Part model, mm, in its own coordinate system. A direction names the side the tool comes from. Coordinates: 2 decimals unless noted, no trailing zeros. Loops run counter-clockwise (first coordinate to the right, second up) from the corner with the lowest first, then second, coordinate; pieces in that order, holes last.
Autodesk Inventor part; units mm, degrees
ref_plane "YZ Plane" through (0, 0, 0) normal (1, 0, 0) x (0, 1, 0)
ref_plane "XZ Plane" through (0, 0, 0) normal (0, 1, 0) x (-1, 0, 0)
ref_plane "XY Plane" through (0, 0, 0) normal (0, 0, 1) x (1, 0, 0)
sketch "Sketch1" plane through (0, 0, 0) normal (0, 0, 1) x (1, 0, 0)
  circle A0 centre (0, 0) radius 9.525
  dimension "d0" = 19.05
extrude "Extrusion1" add sketch "Sketch1" along normal blind 25.4
sketch "Sketch2" plane through (0, 0, 25.4) normal (0, 0, 1) x (1, 0, 0)
  circle A0 centre (0, 0) radius 3.175
  dimension "d3" = 6.35
extrude "Extrusion2" add sketch "Sketch2" along normal blind 25.4
sketch "Sketch3" plane through (0, 0, 50.8) normal (0, 0, 1) x (1, 0, 0)
  line L0 (-0.762, 4.064) -> (0.762, 4.064)
  line L1 (0.762, 4.064) -> (0.762, 2.2428)
  line L2 (0.762, 2.2428) -> (-0.762, 2.2428)
  line L3 (-0.762, 2.2428) -> (-0.762, 4.064)
  point P0 (0, 0)
  dimension "d6" = 4.064
  dimension "d7" = 0.762
  dimension "d8" = 1.524
extrude "Extrusion3" add sketch "Sketch3" against normal blind 12.7
sketch "Sketch4" plane through (0, 0, 0) normal (0, 1, 0) x (-1, 0, 0)
  line L0 (-9.525, 0) -> (-9.525, 25.4)
  line L1 (-9.525, 25.4) -> (-3.175, 25.4)
  line L2 (-3.175, 25.4) -> (-3.175, 50.8)
  line L3 (-3.175, 50.8) -> (3.175, 50.8)
  line L4 (3.175, 50.8) -> (3.175, 25.4)
  line L5 (3.175, 25.4) -> (9.525, 25.4)
  line L6 (9.525, 25.4) -> (9.525, 0)
  line L7 (9.525, 0) -> (-9.525, 0)
  circle A0 centre (0, 12.7) radius 3.175
  point P0 (0, 0)
  dimension "d11" = 6.35
  dimension "d12" = 12.7
  dimension "d13" = 9.525
extrude "Extrusion4" add sketch "Sketch4" along normal blind 76.2 contours A0
sketch "Sketch5" plane through (0, 76.2, 12.7) normal (0, 1, 0) x (1, 0, 0)
  arc A0 (9.525, 0) -> (-9.525, 0) centre (0, 0) ccw
  line L0 (-9.525, 0) -> (9.525, 0)
  line L1 (9.525, 12.7) -> (9.525, -12.7)
  point P0 (0, 12.7)
  dimension "d16" = 19.05
revolve "Revolution1" add sketch "Sketch5" angle 360 about axis through (-9.525, 76.2, 12.7) along (1, 0, 0)
chamfer "Chamfer1" distance 1.524 angle 45 1 edges at (-9.525, 0, 0)
properties part number "Handle" material "Stainless Steel"
Q1. Saw through at B-B (z = 12.7). List the corners of the cut face in (x, y) (3 decimals), plus the area to 3 significant figures.
Q2. Probe line 1 (Z direction, x = -7, y = -2); line 2 (Y direction, x = -4.25, z = 9); line 3 (Y direction, x = 3.5, z = 6.5). List the from-to ranges inside material, lowest first.
Q3. Saw through at A-A (y = 0). List the corners of the cut face in (x, z) (3 decimals), plus the area to 3 significant figures.
Q4. Drop flat-ended pins along their axis: P1, Ø1.5, axis at x = -7, z = 15.5, coming from the +Y side; P2, Ø1.5, axis at x = -2.5, z = 12, coming from the -Y side; P3, Ø0.5, axis at y = 3.5, z = 43.5, coming from the -X side. Give the stop position or say it passes through.
Q5. Saw through at C-C (y = 19.5). List the corners of the cut face in (x, z) (3 decimals), plus the area to 3 significant figures.
Q6. Tool access for faces 1 (the flat face through (0, 0, 0)), 2 (the cylindrical face through (0.69, 37.69, 15.8)): list every direction of +Z, -Z, +X, -X, +Y, -Y with a clear straight run to the whole face (end or side of a thin tool).
Checked values:
1. outline: (-3.175, 8.98) arc R9.525 ccw (long way) to (3.175, 8.98) - (3.175, 67.22) arc R9.525 ccw (long way) to (-3.175, 67.22) - close
1. area: 935 mm2
2. line 1: z = 0 to 25.4
2. line 2: y = -8.52 to 8.52, 68.52 to 83.88
2. line 3: y = -8.86 to 8.86, 69.87 to 82.53
3. outline: (-9.525, 1.524) - (-8.001, 0) - (8.001, 0) - (9.525, 1.524) - (9.525, 25.4) - (3.175, 25.4) - (3.175, 50.8) - (-3.175, 50.8) - (-3.175, 25.4) - (-9.525, 25.4) - close
3. area: 643 mm2
4. P1: stops at y = 82.88
4. P2: stops at y = -9.36
4. P3: stops at x = -0.76
5. outline: circle Ø6.35 at (0, 12.7)
5. area: 31.7 mm2
6. face 1: -Z, +X, -X, +Y, -Y
6. face 2: none
